Could you check a few things on this model? Use its own coordinates, in mm. A direction names the side the tool comes from. Give positions to 0.01 mm unless a question says otherwise; leave off trailing zeros. Order: outer loops, then holes, each group sorted by start corner. A loop starts at its lowest first (then second) coordinate and runs counter-clockwise, first axis right, second up. Notation, with made-up numbers: M -29.5,19.5 L 4.5,19.5 A31 cw 4.5,54.5 Z; hole C -32.5,-32 d5. An arc over 180 degrees is marked long. Use a Markdown table: item, result. Add a question column.
```python
from build123d import *

# Parameters (mm, degrees)
F0_W        = 11
F0_H        = 12.5
F0_R        = 2.5
F1_DEPTH    = 4
F2_R        = 2.5
F3_DEPTH    = 3
F4_W        = 11
F4_H        = 1
F5_DEPTH    = 2
F6_W        = 11
F6_H        = 12.5
F7_DEPTH    = 0.7
F8_DEPTH    = 25
F9_T1_DEPTH = 21.7
F11_DEPTH   = 2
F12_R       = 2.99999


# Not quite as in the source:
# - a fillet or chamfer that OpenCascade refuses, or shapes differently, is made with other operations: its cross-section is extruded or revolved along the edge and cut away or added
# - a fillet or chamfer is up to 0.001 mm smaller than in the source, because OpenCascade refuses the exact size


with BuildPart() as f1:
    # F0 (on Top) → F1 (new body)
    with BuildSketch(Plane.XY):
        Rectangle(F0_W, F0_H)
        Circle(F0_R, mode=Mode.SUBTRACT)
    extrude(amount=-F1_DEPTH)

    # F2 (on Top) → F3 (cut)
    with BuildSketch(Plane.XY):
        Polygon((2.1650635095, 3.75), (-2.1650635095, 3.75), (-4.3301270189, 0), (-2.1650635095, -3.75), (2.1650635095, -3.75), (4.3301270189, 0), align=None)
        Circle(F2_R, mode=Mode.SUBTRACT)
    extrude(amount=-F3_DEPTH, mode=Mode.SUBTRACT)

    # F4 (on face) → F5 (join)
    with BuildSketch(Plane.XY):
        with Locations((0, 5.75)):
            Rectangle(F4_W, F4_H)
        with Locations((0, -5.75)):
            Rectangle(F4_W, F4_H)
    extrude(amount=F5_DEPTH)

    # F6 (on face) → F7 (join)
    with BuildSketch(Plane.XY.offset(2)):
        Rectangle(F6_W, F6_H)
    extrude(amount=F7_DEPTH)

    # F2 (on Top) → F8 (cut)
    with BuildSketch(Plane.XY):
        Polygon((2.1650635095, 3.75), (-2.1650635095, 3.75), (-4.3301270189, 0), (-2.1650635095, -3.75), (2.1650635095, -3.75), (4.3301270189, 0), align=None)
        Circle(F2_R, mode=Mode.SUBTRACT)
        Circle(F2_R)
    extrude(amount=F8_DEPTH, mode=Mode.SUBTRACT)

    # F9: fillet of radius 3 on 4 edges, made by hand

    # F9_s2 → F9_t1 (cut)
    with BuildSketch(Plane.XY.offset(-11.5)):
        with BuildLine():
            ThreePointArc((-2.5, -6.25), (-4.6213203436, -5.3713203436), (-5.5, -3.25))
            Line((-5.5, -3.25), (-5.5, -6.25))
            Line((-5.5, -6.25), (-2.5, -6.25))
        make_face()
        with BuildLine():
            ThreePointArc((2.5, -6.25), (4.6213203436, -5.3713203436), (5.5, -3.25))
            Line((5.5, -3.25), (5.5, -6.25))
            Line((5.5, -6.25), (2.5, -6.25))
        make_face()
        with BuildLine():
            ThreePointArc((5.5, 3.25), (4.6213203436, 5.3713203436), (2.5, 6.25))
            Line((2.5, 6.25), (5.5, 6.25))
            Line((5.5, 6.25), (5.5, 3.25))
        make_face()
        with BuildLine():
            ThreePointArc((-5.5, 3.25), (-4.6213203436, 5.3713203436), (-2.5, 6.25))
            Line((-2.5, 6.25), (-5.5, 6.25))
            Line((-5.5, 6.25), (-5.5, 3.25))
        make_face()
    extrude(amount=F9_T1_DEPTH, mode=Mode.SUBTRACT)

    # F10 (on face) → F11 (cut)
    with BuildSketch(Plane.XY.offset(2.7)):
        Polygon((2.2805335633, 3.95), (-2.2805335633, 3.95), (-4.5610671266, 0), (-2.2805335633, -3.95), (2.2805335633, -3.95), (4.5610671266, 0), align=None)
    extrude(amount=-F11_DEPTH, mode=Mode.SUBTRACT)

    # F12 (radius 3 in the source; OpenCascade refuses exactly that, so slightly less here)
    f12_edges = [f1.edges().sort_by_distance(p)[0] for p in [
        (0, -6.25, -4),
    ]]
    fillet(f12_edges, radius=F12_R)


solid = f1.part
```
1) We'd pull the mould along X, two halves only. Please class faces 4 (the face through (0, 5.25, 1)), 5 (the face through (-0.54, -2.44, -3.49)), 6 (the face through (-5.5, 0, -0.5)): pulls with the +X half, pulls with the -X half, needs draft (parallel to the pull), parting line crosses it, or undercut.
2) Suppose I cut it at D-D on x = 2. Please give me the cut outline in (y, z), and give its area (3 significant figures).
3) Suppose I cut it at B-B on x = 0. Please give me the cut outline in (y, z).
4) Suppose I cut it at A-A on z = 1.25. Please give me the cut outline in (x, y), and give its area (3 significant figures).
5) For pin 1 (2 mm diameter, centred on x = -4, z = -1, fed in from +Y); pin 2 (1 mm diameter, centred on x = -3.5, z = -3, fed in from -Y), each with a flat end and sliding along its axis, tell me the tip position at first contact or that it passes through.
6) Suppose I cut it at C-C on y = 2. Please give me the cut outline in (x, z), and give its area (3 significant figures).
7) Please list where these lines run through material, in increasing order: line 1 (Y direction, x = -2, z = -0.5); line 2 (Y direction, x = 2.5, z = 0.5); line 3 (X direction, y = -2.75, z = -0.25). Write a range as from..to.
8) For faces 1 (the face through (0.04, -5.35, -3.14)), 2 (the face through (-3.437, -1.947, 2.355)), 3 (the face through (-4, 1, 0)), which set-ups out of +Z, -Z, +X, -X, +Y, -Y let a thin tool reach every point of the face, with its end or its side?
Values found:
| question | item | result |
|---|---|---|
| 1 | face 4 | needs draft |
| 1 | face 5 | undercut |
| 1 | face 6 | pulls with the -X half |
| 2 | outline | M -6.25,-1 A3 ccw -3.25,-4 L -1.5,-4 L -1.5,-3 L -3.75,-3 L -3.75,0 L -5.25,0 L -5.25,2 L -3.95,2 L -3.95,2.7 L -6.25,2.7 Z; M 1.5,-4 L 3.25,-4 A3 ccw 6.25,-1 L 6.25,2.7 L 3.95,2.7 L 3.95,2 L 5.25,2 L 5.25,0 L 3.75,0 L 3.75,-3 L 1.5,-3 Z |
| 2 | area | 27.9 mm^2 |
| 3 | outline | M -6.25,-1 A3 ccw -3.25,-4 L -2.5,-4 L -2.5,-3 L -3.75,-3 L -3.75,0 L -5.25,0 L -5.25,2 L -3.95,2 L -3.95,2.7 L -6.25,2.7 Z; M 2.5,-4 L 3.25,-4 A3 ccw 6.25,-1 L 6.25,2.7 L 3.95,2.7 L 3.95,2 L 5.25,2 L 5.25,0 L 3.75,0 L 3.75,-3 L 2.5,-3 Z |
| 4 | outline | M -4.74,-5.25 A3 ccw -2.5,-6.25 L 2.5,-6.25 A3 ccw 4.74,-5.25 Z; M -4.74,5.25 L 4.74,5.25 A3 ccw 2.5,6.25 L -2.5,6.25 A3 ccw Z |
| 4 | area | 16.2 mm^2 |
| 5 | pin 1 | stops at y = 6.21 |
| 5 | pin 2 | stops at y = -5.7 |
| 6 | outline | M -5.5,-1 A3 ccw -2.5,-4 L -1.5,-4 L -1.5,-3 L -3.18,-3 L -3.18,0 L -5.5,0 Z; M -5.5,2 L -3.41,2 L -3.41,2.7 L -5.5,2.7 Z; M 1.5,-4 L 2.5,-4 A3 ccw 5.5,-1 L 5.5,0 L 3.18,0 L 3.18,-3 L 1.5,-3 Z; M 3.41,2 L 5.5,2 L 5.5,2.7 L 3.41,2.7 Z |
| 6 | area | 21.0 mm^2 |
| 7 | line 1 | y = -6.25..-3.75, 3.75..6.25 |
| 7 | line 2 | y = -6.25..-5.25, 5.25..6.25 |
| 7 | line 3 | x = -5.5..-2.74, 2.74..5.5 |
| 8 | face 1 | -Z, +X, -X, -Y |
| 8 | face 2 | +Z |
| 8 | face 3 | +X, -X |
